Work out the finished part from the listing and answer in its coordinate system (mm). A direction names the side the tool comes from. Give positions to 0.01 mm unless a question says otherwise; leave off trailing zeros. Order: outer loops, then holes, each group sorted by start corner. A loop starts at its lowest first (then second) coordinate and runs counter-clockwise, first axis right, second up. Notation, with made-up numbers: M 54,-24 L 81,-24 A23 cw 81,-1 Z; hole C 52,-7.5 d6. An arc over 180 degrees is marked long. One line per item, written item: value.
from build123d import *

# Parameters (mm, degrees)
BOSS_EXTRUDE1_DEPTH   = 10
BOSS_EXTRUDE1_2_DEPTH = 10
BOSS_EXTRUDE1_3_DEPTH = 10
BOSS_EXTRUDE1_4_DEPTH = 10
SKETCH1_3_W           = 20
SKETCH1_3_H           = 20
SKETCH1_3_R           = 2.5
BOSS_EXTRUDE2_DEPTH   = 3
SKETCH3_W             = 4
SKETCH3_H             = 20
BOSS_EXTRUDE3_DEPTH   = 35
BOSS_EXTRUDE4_START   = -188
BOSS_EXTRUDE4_DEPTH   = 38
BOSS_EXTRUDE4_START_2 = -153
BOSS_EXTRUDE4_2_DEPTH = 3
BOSS_EXTRUDE8_START   = -188
BOSS_EXTRUDE8_DEPTH   = 38
BOSS_EXTRUDE8_START_2 = -153
BOSS_EXTRUDE8_2_DEPTH = 3
SKETCH4_R             = 1.3
CUT_EXTRUDE1_DEPTH    = 4
SKETCH5_R             = 2.1
CUT_EXTRUDE2_DEPTH    = 200.679234698


# Read off the part's stored shape, not the designer's step: Boss-Extrude4, Boss-Extrude8
with BuildPart() as part:
    # Sketch1 → Boss-Extrude1 (new body)
    with BuildSketch(Plane.XZ.offset(150)):
        Polygon((111.9, 58), (108.414213562, 58), (112.414213562, 54), (117.585786438, 54), (121.585786438, 58), (118.1, 58), align=None)
    extrude(amount=-BOSS_EXTRUDE1_DEPTH)



with BuildPart() as body_2:
    # Sketch1 → Boss-Extrude1 2 (new body)
    with BuildSketch(Plane.XZ.offset(150)):
        Polygon((111, 47.414213562), (111, 52.585786438), (107, 56.585786438), (107, 53.1), (107, 46.9), (107, 43.414213562), align=None)
    extrude(amount=-BOSS_EXTRUDE1_2_DEPTH)


with BuildPart() as body_3:
    # Sketch1 → Boss-Extrude1 3 (new body)
    with BuildSketch(Plane.XZ.offset(150)):
        Polygon((123, 53.1), (123, 56.585786438), (119, 52.585786438), (119, 47.414213562), (123, 43.414213562), (123, 46.9), align=None)
    extrude(amount=-BOSS_EXTRUDE1_3_DEPTH)


with BuildPart() as body_4:
    # Sketch1 → Boss-Extrude1 4 (new body)
    with BuildSketch(Plane.XZ.offset(150)):
        Polygon((112.414213562, 46), (108.414213562, 42), (111.9, 42), (118.1, 42), (121.585786438, 42), (117.585786438, 46), align=None)
    extrude(amount=-BOSS_EXTRUDE1_4_DEPTH)


with BuildPart() as part_1:
    add(part.part)

    add(body_2.part)  # Boss-Extrude2 merges body 2

    add(body_3.part)  # Boss-Extrude2 merges body 3

    add(body_4.part)  # Boss-Extrude2 merges body 4
    # Sketch1<3> → Boss-Extrude2 (add)
    with BuildSketch(Plane.XZ.offset(150)):
        with Locations((115, 50)):
            Rectangle(SKETCH1_3_W, SKETCH1_3_H)
        with Locations(Location((115, 50, 0), (0, 0, 270))):
            Circle(SKETCH1_3_R, mode=Mode.SUBTRACT)
    extrude(amount=BOSS_EXTRUDE2_DEPTH)

    # Sketch3 → Boss-Extrude3 (add)
    with BuildSketch(Plane.XZ.offset(153)):
        with Locations((107, 50)):
            Rectangle(SKETCH3_W, SKETCH3_H)
    extrude(amount=BOSS_EXTRUDE3_DEPTH)

    # Boss-Extrude4 outline → Boss-Extrude4 (add)
    with BuildSketch(Plane(origin=(0, 0, 0), x_dir=(1, 0, 0), z_dir=(0, 1, 0)).offset(BOSS_EXTRUDE4_START)):
        Polygon((105, -34.641016151), (105, -40), (109, -40), (109, -35.712812921), align=None)
    extrude(amount=BOSS_EXTRUDE4_DEPTH)

    # Boss-Extrude4 2 outline → Boss-Extrude4 2 (add)
    with BuildSketch(Plane(origin=(0, 0, 0), x_dir=(1, 0, 0), z_dir=(0, 1, 0)).offset(BOSS_EXTRUDE4_START_2)):
        Polygon((109, -35.712812921), (109, -40), (125, -40), align=None)
    extrude(amount=BOSS_EXTRUDE4_2_DEPTH)

    # Boss-Extrude8 outline → Boss-Extrude8 (add)
    with BuildSketch(Plane(origin=(0, 0, 0), x_dir=(1, 0, 0), z_dir=(0, 1, 0)).offset(BOSS_EXTRUDE8_START)):
        Polygon((105, -60), (105, -65.358983849), (109, -64.287187079), (109, -60), align=None)
    extrude(amount=BOSS_EXTRUDE8_DEPTH)

    # Boss-Extrude8 2 outline → Boss-Extrude8 2 (add)
    with BuildSketch(Plane(origin=(0, 0, 0), x_dir=(1, 0, 0), z_dir=(0, 1, 0)).offset(BOSS_EXTRUDE8_START_2)):
        Polygon((109, -60), (109, -64.287187079), (125, -60), align=None)
    extrude(amount=BOSS_EXTRUDE8_2_DEPTH)

    # Sketch4 → Cut-Extrude1 (cut)
    with BuildSketch(Plane(origin=(105, 0, -65), x_dir=(0, 0, -1), z_dir=(1, 0, 0))):
        with Locations(Location((-115, -164.5, 0), (0, 0, 180))):
            Circle(SKETCH4_R)
        with Locations(Location((-105.5, -174, 0), (0, 0, 180))):
            Circle(SKETCH4_R)
        with Locations(Location((-115, -183.5, 0), (0, 0, 180))):
            Circle(SKETCH4_R)
        with Locations(Location((-124.5, -174, 0), (0, 0, 180))):
            Circle(SKETCH4_R)
    extrude(amount=CUT_EXTRUDE1_DEPTH, mode=Mode.SUBTRACT)

    # Sketch5 → Cut-Extrude2 (cut, through all)
    with BuildSketch(Plane(origin=(109, 0, 0), x_dir=(0, 0, -1), z_dir=(1, 0, 0))):
        with Locations((-50, -174)):
            Circle(SKETCH5_R)
    extrude(amount=-CUT_EXTRUDE2_DEPTH, mode=Mode.SUBTRACT)


solid = part_1.part
(1) Which of the six approach directions +Z, -Z, +X, -X, +Y, -Y give full straight-line access (tool end or side, diameter ignored) to faces 1 (the flat face through (123, -145, 50)), 2 (the flat face through (119, -153, 50)), 3 (the flat face through (107, -145, 50)), 4 (the flat face through (120.972, -145.07, 45.442))?
Findings:
face 1: +Z, -Z, +X, +Y
face 2: +Z, -Z, +X, -Y
face 3: +Z, -Z, -X, +Y
face 4: +Y
(2) Determine the mould class of faces 5 (the flat face through (115, -140, 56)), 6 (the flat face through (121.028, -145.07, 54.614)), 7 (the cylindrical face through (106.972, -165.379, 49.042)) for opening direction Y: pulls with the +Y half, pulls with the -Y half, needs draft (parallel to the pull), parting line crosses it, or undercut.
Findings:
face 5: pulls with the +Y half
face 6: needs draft
face 7: undercut
(3) Section B-B, the plane y = -164.5 is taken. Give the vertices of the cut face in (x, z), then the cut area to 3 significant figures.
Findings:
outline: M 105,34.64 L 109,35.71 L 109,48.7 L 105,48.7 Z; M 105,51.3 L 109,51.3 L 109,64.29 L 105,65.36 Z
area: 108 mm^2
(4) Section A-A, the plane z = 40.5 is taken. Give the vertices of the cut face in (x, y).
Findings:
outline: M 105,-188 L 109,-188 L 109,-175.3 L 105,-175.3 Z; M 105,-172.7 L 109,-172.7 L 109,-153 L 125,-153 L 125,-150 L 105,-150 Z
(5) Find the intervals of material crossed by probe 1 along Y at (x, z) = (107.3, 50); probe 2 along Y at (x, z) = (106.15, 50); probe 3 along X at (y, z) = (-151, 50), in increasing order. Write a range as from..to.
Findings:
probe 1: y = -188..-184.8, -182.2..-176.1, -171.9..-165.8, -163.2..-140
probe 2: y = -188..-184.8, -182.2..-176.1, -171.9..-165.8, -163.2..-150
probe 3: x = 105..112.5, 117.5..125
(6) Section D-D, the plane z = 50 is taken. Give the number of separate pieces and of enclosed holes in the cut face, then the cut area to 3 significant figures.
Findings:
separate pieces: 5
enclosed holes: 0
area: 227 mm^2
(7) Section C-C, the plane y = -174 is taken. Give the vertices of the cut face in (x, z), then the cut area to 3 significant figures.
Findings:
outline: M 105,34.64 L 109,35.71 L 109,39.2 L 105,39.2 Z; M 105,41.8 L 109,41.8 L 109,47.9 L 105,47.9 Z; M 105,52.1 L 109,52.1 L 109,58.2 L 105,58.2 Z; M 105,60.8 L 109,60.8 L 109,64.29 L 105,65.36 Z
area: 81.0 mm^2
(8) Given P1, Ø1, axis at x = 118, z = 61.5, coming from the +Y side; P2, Ø6, axis at y = -180, z = 38, coming from the +X side; P3, Ø5, axis at y = -146, z = 52, coming from the +X side, each flat-ended and moving along its own axis, determine where each tip first touches the part or whether it passes through.
Findings:
P1: stops at y = -150
P2: stops at x = 109
P3: stops at x = 123
